CAD build for the part. Positions are in the model's coordinates, mm. Face numbers are marked on the shaded views. A direction names the side the tool comes from. Give positions to 0.01 mm unless a question says otherwise; leave off trailing zeros. Loops run counter-clockwise (first coordinate to the right, second up) from the corner with the lowest first, then second, coordinate; pieces in that order, holes last. Notation, with made-up numbers: M 38.5,40.25 L 83.5,40.25 A34 cw 83.5,77.25 Z; hole C 84,41 d9. An arc over 180 degrees is marked long. Answer as CSV lines item,"result".
from build123d import *

# Parameters (mm, degrees)
BOSS_EXTRU_1_DEPTH = 5


with BuildPart() as part:
    # Esquisse1 → Boss.-Extru.1 (new body)
    with BuildSketch(Plane.XY):
        with BuildLine():
            Line((-10, 15), (-10, 8.925037924))
            Line((-10, 8.925037924), (-3.364765454, 3.698425806))
            ThreePointArc((-3.364765454, 3.698425806), (5, 0), (-3.364765454, -3.698425806))
            Line((-3.364765454, -3.698425806), (-10, -8))
            Line((-10, -8), (-10, -15))
            Line((-10, -15), (10, -15))
            Line((10, -15), (10, 15))
            Line((10, 15), (-10, 15))
        make_face()
    extrude(amount=BOSS_EXTRU_1_DEPTH)


solid = part.part
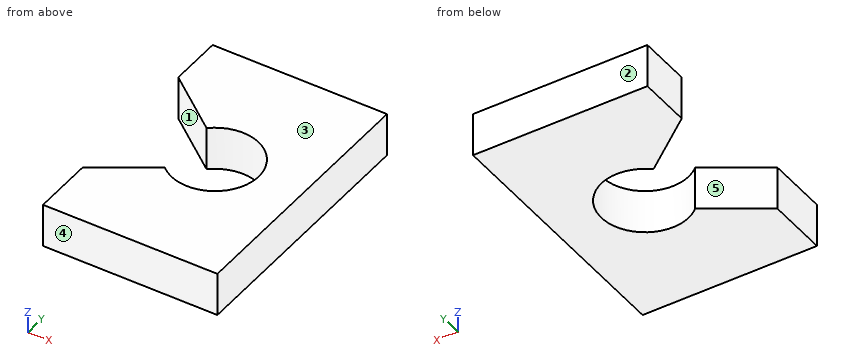
1) Band-saw the part on C-C on x = -4.75. Give the cut face in (y, z).
Answer below:
outline,"M -15,0 L -4.6,0 L -4.6,5 L -15,5 Z; M 4.79,0 L 15,0 L 15,5 L 4.79,5 Z"
2) Flat gauge pins, fed straight in: pin 1 (3 mm diameter, centred on y = 8.5, z = 1.5, fed in from -X); pin 2 (1 mm diameter, centred on y = -1.5, z = 2.5, fed in from -X). Where does each tip first touch, or does it go through?
Answer below:
pin 1,"stops at x = -10"
pin 2,"stops at x = 4.58"
3) Which spindle directions (+Z, -Z, +X, -X, +Y, -Y) get a long thin tool onto all of the face, cutting with end or side? Do the marked faces 1 and 2. Say none if no direction does.
Answer below:
face 1,"+Z, -Z, -X"
face 2,"+Z, -Z, +X, -X, +Y"
4) Band-saw the part on A-A on x = 0. Give the cut face in (y, z), and give its area (4 significant figures).
Answer below:
outline,"M -15,0 L -5,0 L -5,5 L -15,5 Z; M 5,0 L 15,0 L 15,5 L 5,5 Z"
area,"100.0 mm^2"
5) Mould opens along Y. For the marked faces 3, 4 and 5 say: +Y half, -Y half, draft (parallel to the pull), parting line (faces both ways), or undercut.
Answer below:
face 3,"draft"
face 4,"-Y half"
face 5,"undercut"
6) Drill centre lines: line 1 (Y direction, x = 0, z = 1.6); line 2 (X direction, y = 0, z = 3.6); line 3 (Y direction, x = 1.5, z = 3.6). Where is each one in solid material? Low to high. Write a range as from..to.
Answer below:
line 1,"y = -15..-5, 5..15"
line 2,"x = 5..10"
line 3,"y = -15..-4.77, 4.77..15"
7) Band-saw the part on D-D on y = 0. Give the cut face in (x, z), and give its area (3 significant figures).
Answer below:
outline,"M 5,0 L 10,0 L 10,5 L 5,5 Z"
area,"25.0 mm^2"
8) Band-saw the part on B-B on z = 2.15. Give the cut face in (x, y), and give its area (3 significant figures).
Answer below:
outline,"M -10,-15 L 10,-15 L 10,15 L -10,15 L -10,8.93 L -3.36,3.7 A5 cw long -3.36,-3.7 L -10,-8 Z"
area,"449 mm^2"
